Geometry check sheet. Reference: the model listing, model coordinates, mm. Face numbers are marked on the shaded views. A direction names the side the tool comes from. Round coordinates to 2 decimals unless told otherwise and drop trailing zeros. Order: outer loops, then holes, each group sorted by start corner. A loop starts at its lowest first (then second) coordinate and runs counter-clockwise, first axis right, second up. Notation, with made-up numbers: (16, 20.25) - (53, 20.25) arc R24 ccw to (53, 45.25) - close; hole circle Ø10 at (-19.75, 81). An arc over 180 degrees is marked (long way). Return JSON: item names as keys, results as strings. Group by question number.
Q1. Gauge pin test, flat ends, axial feed: pin 1 Ø6.5 at (x, z) = (0, 11.5) entering from +Y; pin 2 Ø1.5 at (x, y) = (-4, 2) entering from +Z; pin 3 Ø1.5 at (y, z) = (-0.5, 2) entering from -X; pin 4 Ø4 at (x, y) = (6.5, -3.5) entering from +Z. Record the tip position at first contact, or that the pin passes through.
Q2. Draft check along Z on the marked faces 1, 2 and 3. Enter one of: pulls with the +Z half, pulls with the -Z half, needs draft (parallel to the pull), parting line crosses it, or undercut.
Q3. Material ranges on line 1 along Z through (x, y) = (-7, -2.75); line 2 along Y through (x, z) = (-2, 13); line 3 along Z through (x, y) = (-11.5, -2), recorded low to high.
Q4. Sectioned sample at A-A, the plane z = 0. Record the cut outline in (x, y), then the cut area to 3 significant figures.
Q5. Tool access check on the marked faces 4 and 5. Record the directions out of +Z, -Z, +X, -X, +Y, -Y that give a thin tool (end or side, any length) a straight path to the whole face; none if there is none.
Q6. Sectioned sample at D-D, the plane z = -11.5. Record the cut outline in (x, y), then the cut area to 3 significant figures.
Q7. Sectioned sample at B-B, the plane x = 11.5. Record the cut outline in (y, z), then the cut area to 3 significant figures.
Q8. Sectioned sample at C-C, the plane y = -1.25. Give the number of separate pieces and of enclosed holes in the cut face, then the cut area to 3 significant figures.
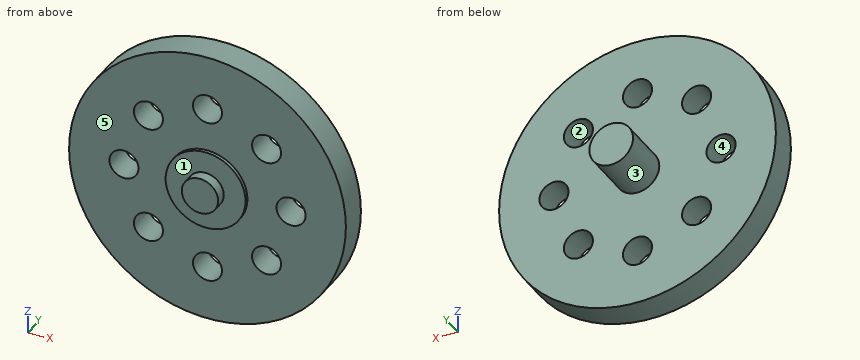
```python
from build123d import *

# Parameters (mm, degrees)
F0_R     = 19.05
F1_DEPTH = 4
F2_R     = 5.5
F2_R_2   = 2.5
F3_DEPTH = 0.5
F4_DEPTH = 1
F5_DEPTH = 1
F6_R     = 3
F7_DEPTH = 7
F8_R     = 2
F9_DEPTH = 25


with BuildPart() as f1:
    # F0 (on Front) → F1 (new body)
    with BuildSketch(Plane.XZ):
        Circle(F0_R)
    extrude(amount=F1_DEPTH)

    # F2 (on face) → F3 (join)
    with BuildSketch(Plane.XZ.offset(4)):
        Circle(F2_R)
        Circle(F2_R_2, mode=Mode.SUBTRACT)
    extrude(amount=F3_DEPTH)

    # F4 (add): a face of the model
    f4_faces = [f1.faces().sort_by_distance(p)[0] for p in [
        (0, -4, 0),
    ]]
    extrude(f4_faces, amount=F4_DEPTH)

    # F5 (add): a face of the model
    f5_faces = [f1.faces().sort_by_distance(p)[0] for p in [
        (0, -5, 0),
    ]]
    extrude(f5_faces, amount=F5_DEPTH)

    # F6 (on face) → F7 (join)
    with BuildSketch(Plane(origin=(0, 0, 0), x_dir=(-1, 0, 0), z_dir=(0, 1, 0))):
        Circle(F6_R)
    extrude(amount=F7_DEPTH)

    # F8 (on face) → F9 (cut)
    with BuildSketch(Plane.XZ.offset(4)):
        with Locations((0, 11.5)):
            Circle(F8_R)
        with Locations((-8.1317279836, 8.1317279836)):
            Circle(F8_R)
        with Locations((-11.5, 0)):
            Circle(F8_R)
        with Locations((-8.1317279836, -8.1317279836)):
            Circle(F8_R)
        with Locations((0, -11.5)):
            Circle(F8_R)
        with Locations((8.1317279836, -8.1317279836)):
            Circle(F8_R)
        with Locations((11.5, 0)):
            Circle(F8_R)
        with Locations((8.1317279836, 8.1317279836)):
            Circle(F8_R)
    extrude(amount=-F9_DEPTH, mode=Mode.SUBTRACT)


solid = f1.part
```
Reply:
{
 "1": {"pin 1": "y = 0", "pin 2": "through", "pin 3": "x = -19.01", "pin 4": "z = 18.51"},
 "2": {"face 1": "needs draft", "face 2": "undercut", "face 3": "parting line crosses it"},
 "3": {"line 1": "-17.72 to -9.78, -6.48 to 6.48, 9.78 to 17.72", "line 2": "-4 to 0", "line 3": "-15.19 to -2, 2 to 15.19"},
 "4": {"outline": "(-19.05, -4) - (-13.5, -4) - (-13.5, 0) - (-19.05, 0) - close; (-9.5, -4) - (-5.5, -4) - (-5.5, -4.5) - (-2.5, -4.5) - (-2.5, -6) - (2.5, -6) - (2.5, -4.5) - (5.5, -4.5) - (5.5, -4) - (9.5, -4) - (9.5, 0) - (3, 0) - (3, 7) - (-3, 7) - (-3, 0) - (-9.5, 0) - close; (13.5, -4) - (19.05, -4) - (19.05, 0) - (13.5, 0) - close", "area": "175 mm^2"},
 "5": {"face 4": "+Y, -Y", "face 5": "-Y"},
 "6": {"outline": "(-15.19, -4) - (-2, -4) - (-2, 0) - (-15.19, 0) - close; (2, -4) - (15.19, -4) - (15.19, 0) - (2, 0) - close", "area": "105 mm^2"},
 "7": {"outline": "(-4, -15.19) - (0, -15.19) - (0, -2) - (-4, -2) - close; (-4, 2) - (0, 2) - (0, 15.19) - (-4, 15.19) - close", "area": "105 mm^2"},
 "8": {"separate pieces": "1", "enclosed holes": "8", "area": "1,040 mm^2"}
}
